```python
from build123d import *

# Parameters (mm, degrees)
F0_R          = 30
F1_DEPTH      = 1500
F2_R          = 29
F3_DEPTH      = 1500
F7_DEPTH      = 150
F7_DEPTH_BACK = 150


# Not quite as in the source:
# - the program builds the solid bodies; features that only make, move or delete a surface that nothing else refers to are left out


with BuildPart() as f1:
    # F0 (on Front) → F1 (new body)
    with BuildSketch(Plane.XZ):
        Circle(F0_R)
    extrude(amount=F1_DEPTH)

    # F2 (on face) → F3 (cut)
    with BuildSketch(Plane.XZ.offset(1500)):
        Circle(F2_R)
    extrude(amount=-F3_DEPTH, mode=Mode.SUBTRACT)

    # F6 (on Right) → F7 (join, two sides)
    with BuildSketch(Plane.YZ) as f7_sk:
        Polygon((-140, 150), (-140, 0), (-140, -150), (360, -150), (360, 150), align=None)
    extrude(amount=F7_DEPTH)
    extrude(f7_sk.sketch, amount=-F7_DEPTH_BACK)


solid = f1.part
```
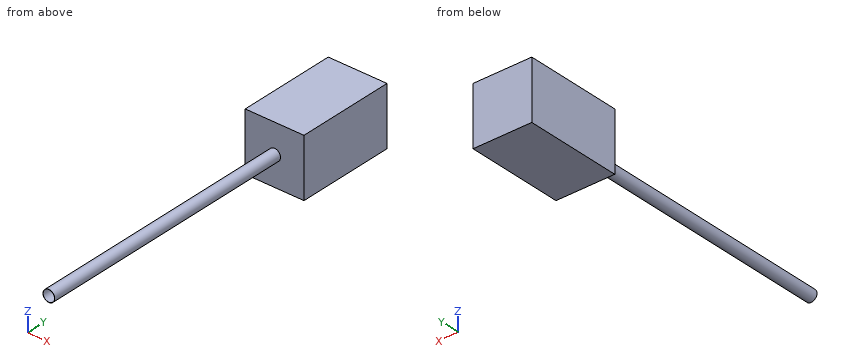
Model file for the job. Use its own axes, mm. Coordinates: 2 decimals unless noted, no trailing zeros. Order: outer loops, then holes, each group sorted by start corner. A loop starts at its lowest first (then second) coordinate and runs counter-clockwise, first axis right, second up. Notation, with made-up numbers: (-21.75, 8.5) -> (6.25, 8.5) arc R22 cw to (6.25, 26.5) -> close; hole circle Ø9 at (-40, 72). An arc over 180 degrees is marked (long way). Answer as a JSON object with one key per item and string values. Group by question number.
1) Cut at C-C, the plane y = -467.5. Write the cut outline in (x, z).
2) Flat gauge pins, fed straight in: pin 1 (6 mm diameter, centred on x = 15.5, y = -278.5, fed in from +Z); pin 2 (8 mm diameter, centred on x = -3, y = -840, fed in from +Z). Where does each tip first touch, or does it go through?
3) Cut at A-A, the plane x = 0. Write the cut outline in (y, z).
4) Drill centre lines: L1, parallel to Z at x = 0, y = -1016; L2, parallel to Y at x = 104, z = -126. Where is each one in solid material? Low to high.
5) Cut at B-B, the plane z = 0. Write the cut outline in (x, y), then the cut area to 3 significant figures.
Check values:
{
 "1": {"outline": "circle Ø60 at (0, 0); hole circle Ø58 at (0, 0)"},
 "2": {"pin 1": "stops at z = 27.27", "pin 2": "stops at z = 30"},
 "3": {"outline": "(-1500, -30) -> (-140, -30) -> (-140, -150) -> (360, -150) -> (360, 150) -> (-140, 150) -> (-140, 30) -> (-1500, 30) -> (-1500, 29) -> (-140, 29) -> (-140, -29) -> (-1500, -29) -> close"},
 "4": {"L1": "z = -30 to -29, 29 to 30", "L2": "y = -140 to 360"},
 "5": {"outline": "(-150, -140) -> (-30, -140) -> (-30, -1500) -> (-29, -1500) -> (-29, -140) -> (29, -140) -> (29, -1500) -> (30, -1500) -> (30, -140) -> (150, -140) -> (150, 360) -> (-150, 360) -> close", "area": "153,000 mm²"}
}
